```python
from build123d import *

# Parameters (mm, degrees)
SKETCH1_R                       = 20
SKETCH1_R_2                     = 1
BOSS_EXTRUDE1_DEPTH             = 21.55
TAP_DRILL_FOR_M5X0_8_TAP1_D     = 4.2
TAP_DRILL_FOR_M5X0_8_TAP1_DEPTH = 5
TAP_DRILL_FOR_M5X0_8_TAP1_TIP   = 1.2618073
SKETCH4_W                       = 6.5
SKETCH4_H                       = 6.5
CUT_EXTRUDE1_DEPTH              = 19.05
CIRPATTERN1_COUNT               = 5
SKETCH5_R                       = 6
SKETCH5_R_2                     = 5
CUT_EXTRUDE2_DEPTH              = 1
FILLET3_R                       = 0.5
CUT_EXTRUDE3_START              = -21.55
SKETCH6_W                       = 8
SKETCH6_H                       = 4.618
SKETCH6_R                       = 2.1
CUT_EXTRUDE3_DEPTH              = 21.55
SKETCH7_R                       = 10.5
CUT_EXTRUDE4_DEPTH              = 6.55
FILLET4_R                       = 2
FILLET5_R                       = 4


# Some blends are built 0.0001 mm under size
with BuildPart() as part:
    # Sketch1 → Boss-Extrude1 (new body)
    with BuildSketch(Plane.XY):
        with Locations((-11.822558412, 14.529752947)):
            Circle(SKETCH1_R)
        with Locations((-11.822558412, 14.529752947)):
            Circle(SKETCH1_R_2, mode=Mode.SUBTRACT)
    extrude(amount=BOSS_EXTRUDE1_DEPTH)

    # Tap Drill for M5x0.8 Tap1
    with Locations(Plane.XY.offset(21.55)):
        with Locations((-11.822558412, 14.529752947)):
            Hole(TAP_DRILL_FOR_M5X0_8_TAP1_D / 2, depth=TAP_DRILL_FOR_M5X0_8_TAP1_DEPTH)
            with Locations((0, 0, -(TAP_DRILL_FOR_M5X0_8_TAP1_DEPTH + TAP_DRILL_FOR_M5X0_8_TAP1_TIP / 2))):  # 118° drill point
                Cone(0, TAP_DRILL_FOR_M5X0_8_TAP1_D / 2, TAP_DRILL_FOR_M5X0_8_TAP1_TIP, mode=Mode.SUBTRACT)

    # Sketch4 → Cut-Extrude1 (cut)
    with BuildSketch(Plane.XY.offset(21.55)):
        with Locations((2.927441588, 14.529752947)):
            Rectangle(SKETCH4_W, SKETCH4_H)
    cut_extrude1 = extrude(amount=-CUT_EXTRUDE1_DEPTH, mode=Mode.SUBTRACT)

    # CirPattern1: Cut-Extrude1 ×5 about axis
    cirpattern1_axis = Axis((-11.822558412, 14.529752947, 0), (0, 0, 1))
    for i in range(1, CIRPATTERN1_COUNT):
        add(cut_extrude1.rotate(cirpattern1_axis, i * 360 / CIRPATTERN1_COUNT), mode=Mode.SUBTRACT)

    # Sketch5 → Cut-Extrude2 (cut)
    with BuildSketch(Plane(origin=(0, 0, 0), x_dir=(-1, 0, 0), z_dir=(0, 0, -1))):
        with Locations((11.822558412, 14.529752947)):
            Circle(SKETCH5_R)
        with Locations((11.822558412, 14.529752947)):
            Circle(SKETCH5_R_2, mode=Mode.SUBTRACT)
    extrude(amount=-CUT_EXTRUDE2_DEPTH, mode=Mode.SUBTRACT)

    # Fillet3
    fillet3_edges = [part.edges().sort_by_distance(p)[0] for p in [
        (-5.822558412, 14.529752947, 1),
        (-6.822558412, 14.529752947, 1),
    ]]
    fillet(fillet3_edges, radius=FILLET3_R - 0.0001)  # a hair under: the kernel refuses the full size

    # Sketch6 → Cut-Extrude3 (cut)
    # profile 1 of 4: a face of its own
    with BuildSketch(Plane.XY.offset(21.55).offset(CUT_EXTRUDE3_START)):
        with Locations((-11.822558412, 14.529752947)):
            Rectangle(SKETCH6_W, SKETCH6_H)
        with Locations((-11.822558412, 14.529752947)):
            Circle(SKETCH6_R, mode=Mode.SUBTRACT)
    # profile 2 of 4: a face of its own
    with BuildSketch(Plane.XY.offset(21.55).offset(CUT_EXTRUDE3_START)):
        with Locations((-11.822558412, 14.529752947)):
            Circle(SKETCH6_R)
    # profile 3 of 4: a face of its own
    with BuildSketch(Plane.XY.offset(21.55).offset(CUT_EXTRUDE3_START)):
        Polygon((-11.822558412, 19.146549298), (-7.822558412, 16.838752947), (-15.822558412, 16.838752947), align=None)
    # profile 4 of 4: a face of its own
    with BuildSketch(Plane.XY.offset(21.55).offset(CUT_EXTRUDE3_START)):
        Polygon((-11.822558412, 9.912956595), (-15.822558412, 12.220752947), (-7.822558412, 12.220752947), align=None)
    extrude(amount=CUT_EXTRUDE3_DEPTH, mode=Mode.SUBTRACT)

    # Sketch7 → Cut-Extrude4 (cut)
    with BuildSketch(Plane.XY.offset(21.55)):
        with Locations((-11.822558412, 14.529752947)):
            Circle(SKETCH7_R)
    extrude(amount=-CUT_EXTRUDE4_DEPTH, mode=Mode.SUBTRACT)

    # Fillet4
    # the kernel refuses this fillet: 2 mm, written as the material it takes off along each edge
    with BuildSketch(Plane(origin=(-11.822558412, 14.529752947, 21.55), x_dir=(1, 0, 0), z_dir=(0, -1, 0))) as fillet4_piece_1:
        with BuildLine():
            CenterArc((10.5 + FILLET4_R, -FILLET4_R), FILLET4_R, 90, 90)
            Line((10.5, -FILLET4_R), (10.5, 0))
            Line((10.5, 0), (10.5 + FILLET4_R, 0))
        make_face()
    revolve(axis=Axis((-11.822558412, 14.529752947, 21.55), (0, 0, 1)), mode=Mode.SUBTRACT)

    # Fillet5
    fillet5_edges = [part.edges().sort_by_distance(p)[0] for p in [
        (-22.322558412, 14.529752947, 15),
    ]]
    fillet(fillet5_edges, radius=FILLET5_R)


solid = part.part
```
For this review, take the finished solid that the model builds, in its own axes (mm). A direction names the side the tool comes from. Round coordinates to 2 decimals unless told otherwise and drop trailing zeros. Loops run counter-clockwise (first coordinate to the right, second up) from the corner with the lowest first, then second, coordinate; pieces in that order, holes last.
Q1. Mouldability with a two-part tool opening along Y and no side actions: class faces 4 (the face through (-3, 24, 21.55)), 5 (the face through (-15.823, 14, 7)), 6 (the face through (-27.694, 2.36, 10.624)) as +Y half, -Y half, draft (parallel to the pull), parting line (faces both ways), or undercut.
Result sheet:
face 4: draft
face 5: undercut
face 6: parting line
Q2. Machinability: for faces 1 (the face through (-10.37, -0.46, 12.16)), 2 (the face through (-10.522, 8.672, 0.247)), 3 (the face through (-13.851, 17.976, 7.395)), which of the approach directions +Z, -Z, +X, -X, +Y, -Y give a long, thin tool a straight path to every point of the face, cutting with its end or side? Answer none if there is none.
Result sheet:
face 1: +Z
face 2: -Z
face 3: +Z, -Z
Q3. Add section B-B on y = 31.5. Write out the cut boundary in (x, z), plus the area to 3 significant figures.
Result sheet:
outline: (-22.41, 0) - (-1.24, 0) - (-1.24, 21.55) - (-5.8, 21.55) - (-5.8, 2.5) - (-9.73, 2.5) - (-9.73, 21.55) - (-22.41, 21.55) - close
area: 381 mm2
Q4. Add section C-C on z = 17. Write out the cut boundary in (x, y), plus the area to 3 significant figures.
Result sheet:
outline: circle Ø40 at (-11.82, 14.53); hole (-28.3, 6.58) - (-24.47, 1.32) - (-19.22, 5.14) - (-23.04, 10.4) - close; hole (-28.3, 22.48) - (-23.04, 18.66) - (-19.22, 23.92) - (-24.47, 27.74) - close; hole circle Ø19.93 at (-11.82, 14.53); hole (-11.36, 2.59) - (-9.35, -3.59) - (-3.17, -1.58) - (-5.18, 4.6) - close; hole (-11.36, 26.47) - (-5.18, 24.46) - (-3.17, 30.64) - (-9.35, 32.65) - close; hole (-0.32, 11.28) - (6.18, 11.28) - (6.18, 17.78) - (-0.32, 17.78) - close
area: 733 mm2
Q5. Add section A-A on x = 2. Write out the cut boundary in (y, z).
Result sheet:
outline: (0.08, 0) - (28.98, 0) - (28.98, 21.55) - (17.78, 21.55) - (17.78, 2.5) - (11.28, 2.5) - (11.28, 21.55) - (0.08, 21.55) - close
Q6. Add section D-D on z = 9. Write out the cut boundary in (x, y).
Result sheet:
outline: circle Ø40 at (-11.82, 14.53); hole (-28.3, 6.58) - (-24.47, 1.32) - (-19.22, 5.14) - (-23.04, 10.4) - close; hole (-28.3, 22.48) - (-23.04, 18.66) - (-19.22, 23.92) - (-24.47, 27.74) - close; hole (-15.82, 12.22) - (-11.82, 9.91) - (-7.82, 12.22) - (-7.82, 16.84) - (-11.82, 19.15) - (-15.82, 16.84) - close; hole (-11.36, 2.59) - (-9.35, -3.59) - (-3.17, -1.58) - (-5.18, 4.6) - close; hole (-11.36, 26.47) - (-5.18, 24.46) - (-3.17, 30.64) - (-9.35, 32.65) - close; hole (-0.32, 11.28) - (6.18, 11.28) - (6.18, 17.78) - (-0.32, 17.78) - close
Q7. Insertion check: pin 1 Ø6 at (y, z) = (28.5, 11) entering from +X; pin 2 Ø10 at (y, z) = (6, 2) entering from -X; pin 3 Ø1.4 at (y, z) = (15.5, 11) entering from -X. Each pin has a flat end and moves straight along its axis. Give the tip position at first contact, or say it passes through.
Result sheet:
pin 1: stops at x = 4.9
pin 2: stops at x = -31.51
pin 3: stops at x = -31.82
Q8. To check wall thickness, follow line 1 along Y through (x, z) = (-27.5, 7); line 2 along Y through (x, z) = (-21, 19); line 3 along X through (y, z) = (27, 11). State the ranges of each line that lie inside material, in increasing order.
Result sheet:
line 1: y = 2.11 to 5.48, 7.16 to 21.9, 23.58 to 26.95
line 2: y = -3.24 to 3.84, 7.6 to 9.43, 19.63 to 21.46, 25.21 to 32.3
line 3: x = -27.46 to -25.01, -23.46 to -11.19, -4.35 to 3.81
